Can you work these out from the drawing? Everything is in mm from the part's minimum corner. Coordinates: 2 decimals unless noted, no trailing zeros. Write each loop counter-clockwise with the first axis right and the second up, starting at its lowest first coordinate (ties: lowest second). Pieces come first, ordered by that corner, then holes.
(1) Thinking about a two-plate mould opening in X: for the marked faces 1, 2 and 3, which applies, released by +X, released by -X, zero draft, split by the parting line, or undercut?
(2) Imagine slicing it at D-D, the plane z = 80. List the corners of the cut face in (x, y) for me.
(3) Imagine slicing it at A-A, the plane z = 10. List the corners of the cut face in (x, y) for me, plus the area to 3 significant figures.
(4) Please list where these lines run through material, in increasing order: probe 1 along X at (y, z) = (10.5, 75); probe 2 along Z at (x, y) = (9.8, 10); probe 3 along X at (y, z) = (14.5, 29.5).
(5) Imagine slicing it at C-C, the plane x = 9.75. List the corners of the cut face in (y, z) for me, plus the area to 3 significant figures.
(6) For pin 1 Ø3 at (x, y) = (4, 14) entering from -Z; pin 2 Ø6 at (y, z) = (10, 66) entering from -X; pin 3 Ø6 at (x, z) = (7.5, 20) entering from -Y, each with a flat end and sliding along its axis, tell me the tip position at first contact or that it passes through.
(7) Imagine slicing it at B-B, the plane y = 10. List the corners of the cut face in (x, z) for me.
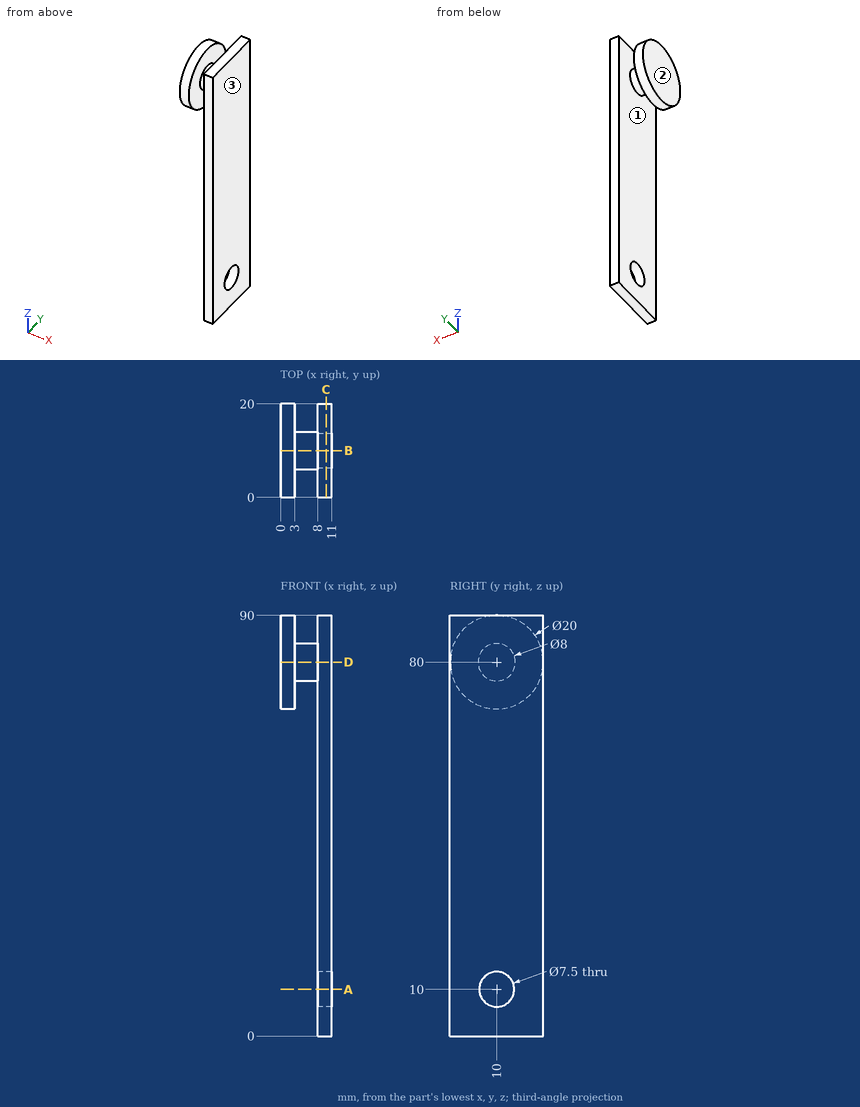
Recorded:
1. face 1: undercut
1. face 2: released by -X
1. face 3: released by +X
2. outline: (0, 0) - (3, 0) - (3, 6) - (8, 6) - (8, 0) - (11, 0) - (11, 20) - (8, 20) - (8, 14) - (3, 14) - (3, 20) - (0, 20) - close
3. outline: (8, 0) - (11, 0) - (11, 6.25) - (8, 6.25) - close; (8, 13.75) - (11, 13.75) - (11, 20) - (8, 20) - close
3. area: 37.5 mm2
4. probe 1: x = 0 to 3, 8 to 11
4. probe 2: z = 0 to 6.25, 13.75 to 90
4. probe 3: x = 8 to 11
5. outline: (0, 0) - (20, 0) - (20, 90) - (0, 90) - close; hole circle Ø7.5 at (10, 10)
5. area: 1,760 mm2
6. pin 1: stops at z = 70.42
6. pin 2: stops at x = 8
6. pin 3: stops at y = 0
7. outline: (0, 70) - (3, 70) - (3, 76) - (8, 76) - (8, 13.75) - (11, 13.75) - (11, 90) - (8, 90) - (8, 84) - (3, 84) - (3, 90) - (0, 90) - close; (8, 0) - (11, 0) - (11, 6.25) - (8, 6.25) - close
